The model under review builds one solid part; all positions refer to its coordinate system, in mm. Coordinates: 2 decimals unless noted, no trailing zeros. Order: outer loops, then holes, each group sorted by start corner. A loop starts at its lowest first (then second) coordinate and runs counter-clockwise, first axis right, second up. Notation, with made-up numbers: M -36.5,9.5 L 13.5,9.5 A29 cw 13.5,41.5 Z; hole C 7,-37.5 d9. An arc over 180 degrees is marked long. Write each question's results on one line, items separated by ' | '.
from build123d import *

# Parameters (mm, degrees)
F0_R     = 53
F0_R_2   = 30
F1_DEPTH = 0.6
F2_R     = 1.25
F3_DEPTH = 25
F5_DEPTH = 25
F7_DEPTH = 2


with BuildPart() as f1:
    # F0 (on Top) → F1 (new body)
    with BuildSketch(Plane.XY):
        Circle(F0_R)
        Circle(F0_R_2, mode=Mode.SUBTRACT)
    extrude(amount=F1_DEPTH)

    # F2 (on face) → F3 (cut)
    with BuildSketch(Plane.XY.offset(0.6)):
        with Locations((0, 35)):
            Circle(F2_R)
        with Locations((35, 0)):
            Circle(F2_R)
        with Locations((0, -35)):
            Circle(F2_R)
        with Locations((-35, 0)):
            Circle(F2_R)
    extrude(amount=-F3_DEPTH, mode=Mode.SUBTRACT)

    # F4 (on face) → F5 (cut)
    with BuildSketch(Plane.XY.offset(0.6)):
        with BuildLine():
            ThreePointArc((2.499305, 52.941038), (0, 53), (-2.499305, 52.941038))
            ThreePointArc((-2.499305, 52.941038), (0, 50.5), (2.499305, 52.941038))
        make_face()
    extrude(amount=-F5_DEPTH, mode=Mode.SUBTRACT)

    # F6 (on face) → F7 (cut)
    with BuildSketch(Plane.XY.offset(0.6)):
        with BuildLine():
            Line((-43.218802, 7.620641), (-37.609581, 6.631584))
            ThreePointArc((-37.609581, 6.631584), (-34.145946, 7.281991), (-31.971682, 10.055504))
            ThreePointArc((-31.971682, 10.055504), (-23.699173, 23.699173), (-10.055504, 31.971682))
            ThreePointArc((-10.055504, 31.971682), (-7.281991, 34.145946), (-6.631584, 37.609581))
            Line((-6.631584, 37.609581), (-7.620641, 43.218802))
            ThreePointArc((-7.620641, 43.218802), (-9.913604, 46.602319), (-13.964743, 47.144664))
            ThreePointArc((-13.964743, 47.144664), (-34.768041, 34.768041), (-47.144664, 13.964743))
            ThreePointArc((-47.144664, 13.964743), (-46.602319, 9.913604), (-43.218802, 7.620641))
        make_face()
        with BuildLine():
            Line((7.620641, 43.218802), (6.631584, 37.609581))
            ThreePointArc((6.631584, 37.609581), (7.281991, 34.145946), (10.055504, 31.971682))
            ThreePointArc((10.055504, 31.971682), (23.699173, 23.699173), (31.971682, 10.055504))
            ThreePointArc((31.971682, 10.055504), (34.145946, 7.281991), (37.609581, 6.631584))
            Line((37.609581, 6.631584), (43.218802, 7.620641))
            ThreePointArc((43.218802, 7.620641), (46.602319, 9.913604), (47.144664, 13.964743))
            ThreePointArc((47.144664, 13.964743), (34.768041, 34.768041), (13.964743, 47.144664))
            ThreePointArc((13.964743, 47.144664), (9.913604, 46.602319), (7.620641, 43.218802))
        make_face()
        with BuildLine():
            ThreePointArc((31.971682, -10.055504), (23.699173, -23.699173), (10.055504, -31.971682))
            ThreePointArc((10.055504, -31.971682), (7.281991, -34.145946), (6.631584, -37.609581))
            Line((6.631584, -37.609581), (7.620641, -43.218802))
            ThreePointArc((7.620641, -43.218802), (9.913604, -46.602319), (13.964743, -47.144664))
            ThreePointArc((13.964743, -47.144664), (34.768041, -34.768041), (47.144664, -13.964743))
            ThreePointArc((47.144664, -13.964743), (46.602319, -9.913604), (43.218802, -7.620641))
            Line((43.218802, -7.620641), (37.609581, -6.631584))
            ThreePointArc((37.609581, -6.631584), (34.145946, -7.281991), (31.971682, -10.055504))
        make_face()
        with BuildLine():
            ThreePointArc((-10.055504, -31.971682), (-23.699173, -23.699173), (-31.971682, -10.055504))
            ThreePointArc((-31.971682, -10.055504), (-34.145946, -7.281991), (-37.609581, -6.631584))
            Line((-37.609581, -6.631584), (-43.218802, -7.620641))
            ThreePointArc((-43.218802, -7.620641), (-46.602319, -9.913604), (-47.144664, -13.964743))
            ThreePointArc((-47.144664, -13.964743), (-34.768041, -34.768041), (-13.964743, -47.144664))
            ThreePointArc((-13.964743, -47.144664), (-9.913604, -46.602319), (-7.620641, -43.218802))
            Line((-7.620641, -43.218802), (-6.631584, -37.609581))
            ThreePointArc((-6.631584, -37.609581), (-7.281991, -34.145946), (-10.055504, -31.971682))
        make_face()
    extrude(amount=-F7_DEPTH, mode=Mode.SUBTRACT)


solid = f1.part
1) Take a section at B-B on y = 0. State the section outline as (x, z) points, plus the area to 3 significant figures.
Solutions:
outline: M -53,0 L -36.25,0 L -36.25,0.6 L -53,0.6 Z; M -33.75,0 L -30,0 L -30,0.6 L -33.75,0.6 Z; M 30,0 L 33.75,0 L 33.75,0.6 L 30,0.6 Z; M 36.25,0 L 53,0 L 53,0.6 L 36.25,0.6 Z | area: 24.6 mm2
2) Take a section at C-C on x = 40.5. State the section outline as (y, z) points, plus the area to 3 significant figures.
Solutions:
outline: M -34.19,0 L -27.88,0 L -27.88,0.6 L -34.19,0.6 Z; M -7.14,0 L 7.14,0 L 7.14,0.6 L -7.14,0.6 Z; M 27.88,0 L 34.19,0 L 34.19,0.6 L 27.88,0.6 Z | area: 16.1 mm2
3) To check wall thickness, follow line 1 along X through (y, z) = (-44, 0.3); line 2 along Y through (x, z) = (8, 0.5); line 3 along X through (y, z) = (-38.5, 0.2). State the ranges of each line that lie inside material, in increasing order.
Solutions:
line 1: -29.55 to -21.95, -7.82 to 7.82, 21.95 to 29.55 | line 2: -52.39 to -44.44, -33.23 to -28.91, 28.91 to 33.23, 44.44 to 52.39 | line 3: -36.42 to -30.58, -6.79 to 6.79, 30.58 to 36.42
4) Take a section at D-D on z = 0.5. Count the separate pieces of the cut face and the enclosed holes in it, plus the area to 3 significant figures.
Solutions:
separate pieces: 1 | enclosed holes: 9 | area: 2,890 mm2
5) Take a section at A-A on x = 0. State the section outline as (y, z) points.
Solutions:
outline: M -53,0 L -36.25,0 L -36.25,0.6 L -53,0.6 Z; M -33.75,0 L -30,0 L -30,0.6 L -33.75,0.6 Z; M 30,0 L 33.75,0 L 33.75,0.6 L 30,0.6 Z; M 36.25,0 L 50.5,0 L 50.5,0.6 L 36.25,0.6 Z
6) The part is to be moulded in two halves that separate along Y. For faces 1 (the cylindrical face through (-2.3, -52.95, 0.3)), 2 (the cylindrical face through (9.86, -46.57, 0.3)), say which applies: pulls with the +Y half, pulls with the -Y half, needs draft (parallel to the pull), parting line crosses it, or undercut.
Solutions:
face 1: parting line crosses it | face 2: undercut
7) For pin 1 (3 mm diameter, centred on x = -25, y = 16, fed in from -Z), flat-tipped, find the tip position at first contact; note if it passes through.
Solutions:
pin 1: z = 0
